```python
from build123d import *

# Parameters (mm, degrees)
RESSALTO_EXTRUS_O1_DEPTH = 175


with BuildPart() as part:
    # Esboço1 → Ressalto-extrusão1 (new, symmetric)
    with BuildSketch(Plane.XY):
        Polygon((-13, -4.05), (-15, -4.05), (-15, -15), (-4.05, -15), (-4.05, -13), (-7.5, -13), (-7.5, -11.627272727), (-4.172727273, -8.3), (4.172727273, -8.3), (7.5, -11.627272727), (7.5, -13), (4.05, -13), (4.05, -15), (15, -15), (15, -4.05), (13, -4.05), (13, -7.5), (11.627272727, -7.5), (8.3, -4.172727273), (8.3, 4.172727273), (11.627272727, 7.5), (13, 7.5), (13, 4.05), (15, 4.05), (15, 15), (4.05, 15), (4.05, 13), (7.5, 13), (7.5, 11.627272727), (4.172727273, 8.3), (-4.172727273, 8.3), (-7.5, 11.627272727), (-7.5, 13), (-4.05, 13), (-4.05, 15), (-15, 15), (-15, 4.05), (-13, 4.05), (-13, 7.5), (-11.627272727, 7.5), (-8.3, 4.172727273), (-8.3, -4.172727273), (-11.627272727, -7.5), (-13, -7.5), align=None)
        with BuildLine():
            Line((-7.239339828, -5.233387445), (-5.125358847, -3.119406464))
            ThreePointArc((-5.125358847, -3.119406464), (-5.566897716, -2.238224702), (-5.858217272, -1.296645823))
            Line((-5.858217272, -1.296645823), (-7.3, -0.859788435))
            Line((-7.3, -0.859788435), (-7.3, 0.859788435))
            Line((-7.3, 0.859788435), (-5.858217272, 1.296645823))
            ThreePointArc((-5.858217272, 1.296645823), (-5.566897716, 2.238224702), (-5.125358847, 3.119406464))
            Line((-5.125358847, 3.119406464), (-7.239339828, 5.233387445))
            Line((-7.239339828, 5.233387445), (-5.233387445, 7.239339828))
            Line((-5.233387445, 7.239339828), (-3.119406464, 5.125358847))
            ThreePointArc((-3.119406464, 5.125358847), (-2.238224702, 5.566897716), (-1.296645823, 5.858217272))
            Line((-1.296645823, 5.858217272), (-0.859788435, 7.3))
            Line((-0.859788435, 7.3), (0.859788435, 7.3))
            Line((0.859788435, 7.3), (1.296645823, 5.858217272))
            ThreePointArc((1.296645823, 5.858217272), (2.238224702, 5.566897716), (3.119406464, 5.125358847))
            Line((3.119406464, 5.125358847), (5.233387445, 7.239339828))
            Line((5.233387445, 7.239339828), (7.239339828, 5.233387445))
            Line((7.239339828, 5.233387445), (5.125358847, 3.119406464))
            ThreePointArc((5.125358847, 3.119406464), (5.566897716, 2.238224702), (5.858217272, 1.296645823))
            Line((5.858217272, 1.296645823), (7.3, 0.859788435))
            Line((7.3, 0.859788435), (7.3, -0.859788435))
            Line((7.3, -0.859788435), (5.858217272, -1.296645823))
            ThreePointArc((5.858217272, -1.296645823), (5.566897716, -2.238224702), (5.125358847, -3.119406464))
            Line((5.125358847, -3.119406464), (7.239339828, -5.233387445))
            Line((7.239339828, -5.233387445), (5.233387445, -7.239339828))
            Line((5.233387445, -7.239339828), (3.119406464, -5.125358847))
            ThreePointArc((3.119406464, -5.125358847), (2.238224702, -5.566897716), (1.296645823, -5.858217272))
            Line((1.296645823, -5.858217272), (0.859788435, -7.3))
            Line((0.859788435, -7.3), (-0.859788435, -7.3))
            Line((-0.859788435, -7.3), (-1.296645823, -5.858217272))
            ThreePointArc((-1.296645823, -5.858217272), (-2.238224702, -5.566897716), (-3.119406464, -5.125358847))
            Line((-3.119406464, -5.125358847), (-5.233387445, -7.239339828))
            Line((-5.233387445, -7.239339828), (-7.239339828, -5.233387445))
        make_face(mode=Mode.SUBTRACT)
        Polygon((-11.005952384, -9), (-13, -9), (-13, -13), (-9, -13), (-9, -11.005952384), (-6.294047616, -8.3), (-8.3, -6.294047616), align=None, mode=Mode.SUBTRACT)
        Polygon((9, -11.005952384), (9, -13), (13, -13), (13, -9), (11.005952384, -9), (8.3, -6.294047616), (6.294047616, -8.3), align=None, mode=Mode.SUBTRACT)
        Polygon((11.005952384, 9), (13, 9), (13, 13), (9, 13), (9, 11.005952384), (6.294047616, 8.3), (8.3, 6.294047616), align=None, mode=Mode.SUBTRACT)
        Polygon((-9, 11.005952384), (-9, 13), (-13, 13), (-13, 9), (-11.005952384, 9), (-8.3, 6.294047616), (-6.294047616, 8.3), align=None, mode=Mode.SUBTRACT)
    extrude(amount=RESSALTO_EXTRUS_O1_DEPTH, both=True)


solid = part.part
```
CAD build for the part. Positions are in the model's coordinates, mm. Coordinates: 2 decimals unless noted, no trailing zeros. Return JSON: item names as keys, results as strings. Group by question number.
Q1. Flat gauge pins, fed straight in: pin 1 (1.4 mm diameter, centred on y = 0, z = 63.5, fed in from -X); pin 2 (0.5 mm diameter, centred on y = 0, z = 50.5, fed in from +X); pin 3 (2 mm diameter, centred on x = -3, z = -45, fed in from +Y). Where does each tip first touch, or does it go through?
Q2. Drill centre lines: line 1 (Y direction, x = 12.5, z = 100); line 2 (X direction, y = -5, z = -55.5); line 3 (Y direction, x = -10.75, z = 7.5). Where is each one in solid material? Low to high.
Q3. Pull direction X, two halves, no side cores. Call faces 1 (the face through (0, 8.3, 2)), 2 (the face through (-15, -9, 2)), 3 (the face through (6.5, 3.5, 175)), 4 (the face through (0, -8.3, 2)): released by +X, released by -X, zero draft, split by the parting line, or undercut.
Q4. Cut at A-A, the plane z = 5. State how many separate pieces and enclosed holes the cut face has, then the cut area to 3 significant figures.
Returned:
{
 "1": {"pin 1": "stops at x = -8.3", "pin 2": "stops at x = 8.3", "pin 3": "stops at y = 8.3"},
 "2": {"line 1": "y = -15 to -13, -9 to -7.5, 7.5 to 9, 13 to 15", "line 2": "x = -15 to -13, -9.13 to -7.01, 7.01 to 9.13, 13 to 15", "line 3": "y = -15 to -13, -8.74 to -6.62, 6.62 to 8.74, 13 to 15"},
 "3": {"face 1": "undercut", "face 2": "released by -X", "face 3": "zero draft", "face 4": "undercut"},
 "4": {"separate pieces": "1", "enclosed holes": "5", "area": "341 mm2"}
}
